from build123d import *

# Parameters (mm, degrees)
SKETCH1_W           = 120
SKETCH1_H           = 58
BOSS_EXTRUDE5_DEPTH = 5
SKETCH5_R           = 2.5
CUT_EXTRUDE2_DEPTH  = 5
SKETCH6_W           = 40
SKETCH6_H           = 6
BOSS_EXTRUDE6_DEPTH = 3
SKETCH7_R           = 11.25
CUT_EXTRUDE3_DEPTH  = 2
SKETCH8_R           = 4
CUT_EXTRUDE4_DEPTH  = 12
SKETCH9_R           = 5.1
CUT_EXTRUDE5_DEPTH  = 1.5
SKETCH10_R          = 1.75
CUT_EXTRUDE6_DEPTH  = 21.5


with BuildPart() as part:
    # Sketch1 → Boss-Extrude5 (new body)
    with BuildSketch(Plane(origin=(0, 0, 0), x_dir=(1, 0, 0), z_dir=(0, 1, 0))):
        with Locations((60, 29)):
            Rectangle(SKETCH1_W, SKETCH1_H)
    extrude(amount=BOSS_EXTRUDE5_DEPTH)

    # Sketch5 → Cut-Extrude2 (cut)
    with BuildSketch(Plane(origin=(0, 5, 0), x_dir=(1, 0, 0), z_dir=(0, 1, 0))):
        with Locations(Location((10, 48, 0), (0, 0, 270))):
            Circle(SKETCH5_R)
        with Locations(Location((60, 48, 0), (0, 0, 270))):
            Circle(SKETCH5_R)
        with Locations(Location((110, 48, 0), (0, 0, 270))):
            Circle(SKETCH5_R)
    extrude(amount=-CUT_EXTRUDE2_DEPTH, mode=Mode.SUBTRACT)

    # Sketch6 → Boss-Extrude6 (add)
    with BuildSketch(Plane(origin=(0, 5, 0), x_dir=(1, 0, 0), z_dir=(0, 1, 0))):
        with Locations((35, 48)):
            Rectangle(SKETCH6_W, SKETCH6_H)
        with Locations((85, 48)):
            Rectangle(SKETCH6_W, SKETCH6_H)
    extrude(amount=BOSS_EXTRUDE6_DEPTH)

    # Sketch7 → Cut-Extrude3 (cut)
    with BuildSketch(Plane(origin=(0, 5, 0), x_dir=(1, 0, 0), z_dir=(0, 1, 0))):
        with Locations(Location((60, 13.85, 0), (0, 0, 270))):
            Circle(SKETCH7_R)
    extrude(amount=-CUT_EXTRUDE3_DEPTH, mode=Mode.SUBTRACT)

    # Sketch8 → Cut-Extrude4 (cut)
    with BuildSketch(Plane(origin=(0, 3, 0), x_dir=(1, 0, 0), z_dir=(0, 1, 0))):
        with Locations(Location((60, 13.85, 0), (0, 0, 270))):
            Circle(SKETCH8_R)
    extrude(amount=-CUT_EXTRUDE4_DEPTH, mode=Mode.SUBTRACT)

    # Sketch9 → Cut-Extrude5 (cut)
    with BuildSketch(Plane(origin=(0, 3, 0), x_dir=(1, 0, 0), z_dir=(0, 1, 0))):
        with Locations(Location((60, 13.85, 0), (0, 0, 270))):
            Circle(SKETCH9_R)
    extrude(amount=-CUT_EXTRUDE5_DEPTH, mode=Mode.SUBTRACT)

    # Sketch10 → Cut-Extrude6 (cut)
    with BuildSketch(Plane(origin=(0, 3, 0), x_dir=(1, 0, 0), z_dir=(0, 1, 0))):
        with Locations(Location((52, 13.85, 0), (0, 0, 270))):
            Circle(SKETCH10_R)
        with Locations(Location((60, 21.85, 0), (0, 0, 270))):
            Circle(SKETCH10_R)
        with Locations(Location((68, 13.85, 0), (0, 0, 270))):
            Circle(SKETCH10_R)
        with Locations(Location((60, 5.85, 0), (0, 0, 270))):
            Circle(SKETCH10_R)
    extrude(amount=-CUT_EXTRUDE6_DEPTH, mode=Mode.SUBTRACT)


solid = part.part
Geometry check sheet. Reference: the model listing, model coordinates, mm. A direction names the side the tool comes from. Round coordinates to 2 decimals unless told otherwise and drop trailing zeros. Loops run counter-clockwise (first coordinate to the right, second up) from the corner with the lowest first, then second, coordinate; pieces in that order, holes last.
Item 1: Mould release check, pull along X, two halves, no side actions. Record for faces 4 (the flat face through (120, 2, -29)), 5 (the flat face through (55, 6, -48)), 6 (the flat face through (35, 6, -51)): pulls with the +X half, pulls with the -X half, needs draft (parallel to the pull), parting line crosses it, or undercut.
Item 2: Access from +Z, -Z, +X, -X, +Y, -Y to the whole of each face (thin tool, end or side, straight path). Record for faces 1 (the flat face through (85, 6, -51)), 2 (the flat face through (85, 6, -45)), 3 (the cylindrical face through (65.057, 2.26, -14.514)).
Item 3: Cross-section at B-B on x = 60. Record the boundary of the cut face in (y, z), then the cut area to 3 significant figures.
Item 4: Cross-section at C-C on x = 28.5. Record the boundary of the cut face in (y, z), then the cut area to 3 significant figures.
Item 5: Cross-section at A-A on z = -13.85. Record the boundary of the cut face in (x, y), then the cut area to 3 significant figures.
Item 6: Gauge pin test, flat ends, axial feed: pin 1 (11 mm diameter, centred on x = 63.5, z = -14, fed in from +Y); pin 2 (4 mm diameter, centred on x = 86, z = -22.5, fed in from +Y); pin 3 (2.5 mm diameter, centred on y = 6.5, z = -46.5, fed in from +X). Record the tip position at first contact, or that the pin passes through.
Item 7: Cross-section at D-D on z = -48. Record the boundary of the cut face in (x, y).
Item 8: Thickness scan on line 1 (X direction, y = 2.5, z = -13.85); line 2 (X direction, y = 2.55, z = -48); line 3 (X direction, y = 6, z = -46.5). Record the ranges inside material, lowest first.
Answer sheet:
1. face 4: pulls with the +X half
1. face 5: undercut
1. face 6: needs draft
2. face 1: -Z, +X, -X, +Y
2. face 2: +Z, +X, -X, +Y
2. face 3: +Y
3. outline: (0, -58) - (5, -58) - (5, -50.5) - (0, -50.5) - close; (0, -45.5) - (5, -45.5) - (5, -25.1) - (3, -25.1) - (3, -23.6) - (0, -23.6) - close; (0, -20.1) - (3, -20.1) - (3, -18.95) - (1.5, -18.95) - (1.5, -17.85) - (0, -17.85) - close; (0, -9.85) - (1.5, -9.85) - (1.5, -8.75) - (3, -8.75) - (3, -7.6) - (0, -7.6) - close; (0, -4.1) - (3, -4.1) - (3, -2.6) - (5, -2.6) - (5, 0) - (0, 0) - close
3. area: 172 mm2
4. outline: (0, -58) - (5, -58) - (5, -51) - (8, -51) - (8, -45) - (5, -45) - (5, 0) - (0, 0) - close
4. area: 308 mm2
5. outline: (0, 0) - (50.25, 0) - (50.25, 3) - (48.75, 3) - (48.75, 5) - (0, 5) - close; (53.75, 0) - (56, 0) - (56, 1.5) - (54.9, 1.5) - (54.9, 3) - (53.75, 3) - close; (64, 0) - (66.25, 0) - (66.25, 3) - (65.1, 3) - (65.1, 1.5) - (64, 1.5) - close; (69.75, 0) - (120, 0) - (120, 5) - (71.25, 5) - (71.25, 3) - (69.75, 3) - close
5. area: 507 mm2
6. pin 1: stops at y = 3
6. pin 2: stops at y = 5
6. pin 3: stops at x = 105
7. outline: (0, 0) - (7.5, 0) - (7.5, 5) - (0, 5) - close; (12.5, 0) - (57.5, 0) - (57.5, 5) - (55, 5) - (55, 8) - (15, 8) - (15, 5) - (12.5, 5) - close; (62.5, 0) - (107.5, 0) - (107.5, 5) - (105, 5) - (105, 8) - (65, 8) - (65, 5) - (62.5, 5) - close; (112.5, 0) - (120, 0) - (120, 5) - (112.5, 5) - close
8. line 1: x = 0 to 50.25, 53.75 to 54.9, 65.1 to 66.25, 69.75 to 120
8. line 2: x = 0 to 7.5, 12.5 to 57.5, 62.5 to 107.5, 112.5 to 120
8. line 3: x = 15 to 55, 65 to 105
